```python
from build123d import *

# Parameters (mm, degrees)
F2_R     = 4.7625
F3_DEPTH = 9.525
F6_D     = 3.175
F6_DEPTH = 22.225
F6_START = 0.6225488
F6_TIP   = 0.9538662327
F7_SIZE  = 5.08


# Not quite as in the source:
# - a fillet or chamfer that OpenCascade refuses, or shapes differently, is made with other operations: its cross-section is extruded or revolved along the edge and cut away or added


with BuildPart() as f1:
    # F0 (on Front) → F1 (revolve)
    with BuildSketch(Plane.XZ):
        Polygon((5.470779, 56.2707707286), (0, 56.2707707286), (0, 0), (25.409779, 9.9646151066), (25.409779, 17.1938474178), (31.759779, 17.1938474178), (31.759779, 36.2438474178), (25.409779, 36.2438474178), (25.409779, 48.9438474178), (5.470779, 48.9438474178), align=None)
    revolve(axis=Axis((0, 0, 28.1353853643), (0, 0, -1)))

    # F2 (on face) → F3 (cut)
    with BuildSketch(Plane.XY.offset(56.2707707286)):
        Circle(F2_R)
    extrude(amount=-F3_DEPTH, mode=Mode.SUBTRACT)

    # F4: chamfer of 5.08 on 1 edges, made by hand

    # F4_s1 → F4_t2 (revolve, cut)
    with BuildSketch(Plane.XZ):
        Polygon((0.390779, 56.2707707286), (5.470779, 51.1907707286), (5.470779, 56.2707707286), align=None)
    revolve(axis=Axis((0, 0, 56.2707707286), (0, 0, -1)), mode=Mode.SUBTRACT)

    # F6
    # its depths count from where the whole tool has entered the part; down to there all is cleared
    with Locations(Plane(origin=(0, 0, 0), x_dir=(1, 0, 0), z_dir=(0, 0, -1)).offset(-F6_START)):
        with Locations((0, 0)):
            Hole(F6_D / 2, depth=F6_DEPTH)
            with Locations((0, 0, -(F6_DEPTH + F6_TIP / 2))):  # 118° drill point
                Cone(0, F6_D / 2, F6_TIP, mode=Mode.SUBTRACT)

    # F7
    f7_edges = [f1.edges().sort_by_distance(p)[0] for p in [
        (-25.409779, 0, 36.243847),
        (-25.409779, 0, 48.943847),
        (25.409779, 0, 42.593847),
    ]]
    chamfer(f7_edges, length=F7_SIZE)


solid = f1.part
```
Source: CAD feature listing. Evaluate the final solid. Frame: model axes, mm. A direction names the side the tool comes from. Round coordinates to 2 decimals unless told otherwise and drop trailing zeros. Loops run counter-clockwise (first coordinate to the right, second up) from the corner with the lowest first, then second, coordinate; pieces in that order, holes last. Notation, with made-up numbers: M 86,10.5 L 112,10.5 A12 ccw 112,27.5 Z; hole C -11.75,-34 d11. An arc over 180 degrees is marked long. Use a Markdown table: item, result. Add a question column.
1. Mould query, pull axis Y, two halves, no side actions, for faces 4 (the flat face through (0, 0, 46.746)), 5 (the flat face through (-11.9, -28.4, 36.244)), 6 (the cylindrical face through (24.236, -7.632, 13.63)). Classes: pulls with the +Y half, pulls with the -Y half, needs draft (parallel to the pull), parting line crosses it, or undercut.
2. Contact query for flat-ended pins moving along their axis: P1, Ø6, axis at x = -1, z = 45, coming from the -Y side; P2, Ø8.5, axis at x = 0, y = 0, coming from the +Z side; P3, Ø12, axis at x = 19, y = 4, coming from the +Z side; P4, Ø10.5, axis at x = -2, y = 2, coming from the +Z side. Output: stop coordinate, or through.
3. Section query A-A on z = 25. Return the cut outline in (x, y).
4. Reachability of faces 1 (the cylindrical face through (-6.9, 31, 26.9)), 2 (the flat face through (14.3, -21.3, 17.194)), 3 (the cylindrical face through (-3.78, -2.9, 49.36)) from +Z, -Z, +X, -X, +Y, -Y: full face, straight path, thin tool, end or side. Return the list, or none.
5. Line query: line 1 (Y direction, x = 0, z = 15.25); line 2 (Z direction, x = -19.5, y = 24); line 3 (Y direction, x = 0, z = 50.1). Output: solid intervals per line, ascending.
6. Section query B-B on z = 13.5. Return the cut outline in (x, y) (1 decimal).
Reported:
| question | item | result |
|---|---|---|
| 1 | face 4 | undercut |
| 1 | face 5 | needs draft |
| 1 | face 6 | parting line crosses it |
| 2 | P1 | stops at y = -25.41 |
| 2 | P2 | stops at z = 46.75 |
| 2 | P3 | stops at z = 48.94 |
| 2 | P4 | stops at z = 51.9 |
| 3 | outline | C 0,0 d63.52 |
| 4 | face 1 | +Z, -Z |
| 4 | face 2 | -Z |
| 4 | face 3 | +Z |
| 5 | line 1 | y = -25.41 to -1.59, 1.59 to 25.41 |
| 5 | line 2 | z = 17.19 to 36.24 |
| 5 | line 3 | y = -5.47 to -4.76, 4.76 to 5.47 |
| 6 | outline | C 0,0 d50.8; hole C 0,0 d3.2 |
